Here's how the part is built. I have some questions about the finished solid (model axes, mm). A direction names the side the tool comes from. Give positions to 0.01 mm unless a question says otherwise; leave off trailing zeros. Loops run counter-clockwise (first coordinate to the right, second up) from the corner with the lowest first, then second, coordinate; pieces in that order, holes last.
Q1. For faces 4 (the face through (5, 30, 10)), 5 (the face through (35.436, 3.993, 11.892)), 6 (the face through (11, 20, 10)), which set-ups out of +Z, -Z, +X, -X, +Y, -Y let a thin tool reach every point of the face, with its end or its side?
Q2. Suppose I cut it at B-B (z = 4.5). List the corners of the cut face in (x, y) for me, and give its area (3 significant figures).
Q3. Suppose I cut it at D-D (y = 3.25). List the corners of the cut face in (x, z) for me, and give its area (3 significant figures).
Q4. I need wall thicknesses on probe 1 along Y at (x, z) = (2.5, 15); probe 2 along Z at (x, y) = (37.5, 1.5); probe 3 along X at (y, z) = (22, 4.75). Which ranges of each line are inside material? Lowest first, please.
Q5. Suppose I cut it at A-A (y = 25.1). List the corners of the cut face in (x, z) for me, and give its area (3 significant figures).
Q6. I'm going to push flat-ended pins straight in: P1, Ø3, axis at y = 25.1, z = 15, coming from the +X side; P2, Ø3, axis at x = 20.5, z = 2, coming from the +Y side. Where does each tip first touch, or does it pass through?
Q7. Thinking about a two-plate mould opening in X: for faces 1 (the face through (17, 8.1, 10)), 2 (the face through (5.58, 14.91, 16.03)), 3 (the face through (0, 15, 10)), which applies, pulls with the +X half, pulls with the -X half, needs draft (parallel to the pull), parting line crosses it, or undercut?
Q8. Suppose I cut it at C-C (x = 4). List the corners of the cut face in (y, z) for me, and give its area (3 significant figures).
```python
from build123d import *

# Parameters (mm, degrees)
BOSS_EXTRU_1_DEPTH      = 20
ESQUISSE2_R             = 2.8
ENL_V_MAT_EXTRU_1_DEPTH = 8.1
ENL_V_MAT_EXTRU_2_REACH = 13
ESQUISSE3_R             = 1.3


with BuildPart() as part:
    # Esquisse1 → Boss.-Extru.1 (new body)
    with BuildSketch(Plane.XY):
        Polygon((0, 0), (0, 30), (11, 30), (11, 10), (45, 10), (45, 0), align=None)
    extrude(amount=BOSS_EXTRU_1_DEPTH)

    # Esquisse2 → Enlèv. mat.-Extru.1 (cut)
    with BuildSketch(Plane.XZ):
        with Locations((17.5, 10)):
            Circle(ESQUISSE2_R)
        with Locations((37.5, 10)):
            Circle(ESQUISSE2_R)
    extrude(amount=-ENL_V_MAT_EXTRU_1_DEPTH, mode=Mode.SUBTRACT)

    # Esquisse3 → Enlèv. mat.-Extru.2 (cut, up to next)
    with BuildSketch(Plane(origin=(11, 0, 0), x_dir=(0, 0, -1), z_dir=(1, 0, 0)), mode=Mode.PRIVATE) as enl_v_mat_extru_2_sk1:
        with Locations((-15, 25.1)):
            Circle(ESQUISSE3_R)
    enl_v_mat_extru_2_tool1 = extrude(enl_v_mat_extru_2_sk1.sketch, amount=-ENL_V_MAT_EXTRU_2_REACH, mode=Mode.PRIVATE) & part.part
    add(enl_v_mat_extru_2_tool1.solids().sort_by_distance((11, 25.1, 15))[0], mode=Mode.SUBTRACT)
    # Esquisse3 → Enlèv. mat.-Extru.2 (cut, up to next)
    with BuildSketch(Plane(origin=(11, 0, 0), x_dir=(0, 0, -1), z_dir=(1, 0, 0)), mode=Mode.PRIVATE) as enl_v_mat_extru_2_sk2:
        with Locations((-5, 25.1)):
            Circle(ESQUISSE3_R)
    enl_v_mat_extru_2_tool2 = extrude(enl_v_mat_extru_2_sk2.sketch, amount=-ENL_V_MAT_EXTRU_2_REACH, mode=Mode.PRIVATE) & part.part
    add(enl_v_mat_extru_2_tool2.solids().sort_by_distance((11, 25.1, 5))[0], mode=Mode.SUBTRACT)
    # Esquisse3 → Enlèv. mat.-Extru.2 (cut, up to next)
    with BuildSketch(Plane(origin=(11, 0, 0), x_dir=(0, 0, -1), z_dir=(1, 0, 0)), mode=Mode.PRIVATE) as enl_v_mat_extru_2_sk3:
        with Locations((-5, 15.7)):
            Circle(ESQUISSE3_R)
    enl_v_mat_extru_2_tool3 = extrude(enl_v_mat_extru_2_sk3.sketch, amount=-ENL_V_MAT_EXTRU_2_REACH, mode=Mode.PRIVATE) & part.part
    add(enl_v_mat_extru_2_tool3.solids().sort_by_distance((11, 15.7, 5))[0], mode=Mode.SUBTRACT)
    # Esquisse3 → Enlèv. mat.-Extru.2 (cut, up to next)
    with BuildSketch(Plane(origin=(11, 0, 0), x_dir=(0, 0, -1), z_dir=(1, 0, 0)), mode=Mode.PRIVATE) as enl_v_mat_extru_2_sk4:
        with Locations((-15, 15.7)):
            Circle(ESQUISSE3_R)
    enl_v_mat_extru_2_tool4 = extrude(enl_v_mat_extru_2_sk4.sketch, amount=-ENL_V_MAT_EXTRU_2_REACH, mode=Mode.PRIVATE) & part.part
    add(enl_v_mat_extru_2_tool4.solids().sort_by_distance((11, 15.7, 15))[0], mode=Mode.SUBTRACT)


solid = part.part
```
Solutions:
1. face 4: +Z, -Z, +X, -X, +Y
1. face 5: -Y
1. face 6: +Z, -Z, +X, +Y
2. outline: (0, 0) - (45, 0) - (45, 10) - (11, 10) - (11, 14.5) - (0, 14.5) - close; (0, 16.9) - (11, 16.9) - (11, 23.9) - (0, 23.9) - close; (0, 26.3) - (11, 26.3) - (11, 30) - (0, 30) - close
2. area: 617 mm2
3. outline: (0, 0) - (45, 0) - (45, 20) - (0, 20) - close; hole circle Ø5.6 at (17.5, 10); hole circle Ø5.6 at (37.5, 10)
3. area: 851 mm2
4. probe 1: y = 0 to 14.4, 17 to 23.8, 26.4 to 30
4. probe 2: z = 0 to 7.2, 12.8 to 20
4. probe 3: x = 0 to 11
5. outline: (0, 0) - (11, 0) - (11, 3.7) - (0, 3.7) - close; (0, 6.3) - (11, 6.3) - (11, 13.7) - (0, 13.7) - close; (0, 16.3) - (11, 16.3) - (11, 20) - (0, 20) - close
5. area: 163 mm2
6. P1: stops at x = 11
6. P2: stops at y = 10
7. face 1: undercut
7. face 2: needs draft
7. face 3: pulls with the -X half
8. outline: (0, 0) - (30, 0) - (30, 20) - (0, 20) - close; hole circle Ø2.6 at (15.7, 5); hole circle Ø2.6 at (15.7, 15); hole circle Ø2.6 at (25.1, 5); hole circle Ø2.6 at (25.1, 15)
8. area: 579 mm2
